Build history of the part. All positions in model axes, mm. A direction names the side the tool comes from. Give positions to 0.01 mm unless a question says otherwise; leave off trailing zeros. Loops run counter-clockwise (first coordinate to the right, second up) from the corner with the lowest first, then second, coordinate; pieces in that order, holes last. Notation, with made-up numbers: (-3.5, 39) - (28.5, 39) arc R31 ccw to (28.5, 66) - close; hole circle Ø8 at (22, 8.25). An arc over 180 degrees is marked (long way). Return JSON: item names as keys, results as strings. Group by question number.
1) Slice it at B-B (x = 40). List the corners of the cut face in (y, z).
2) Slice it at A-A (z = 1). Count the separate pieces of the cut face and the enclosed holes in it, and give its area (3 significant figures).
3) Drill centre lines: probe 1 along X at (y, z) = (-6.5, -0.5); probe 2 along Y at (x, z) = (36, 2.25); probe 3 along Y at (x, z) = (6.5, 1.75). Where is each one in solid material? Low to high. Write a range as from..to.
4) Drop flat-ended pins along their axis: pin 1 (4.5 mm diameter, centred on x = 20.5, y = 0.5, fed in from -Z); pin 2 (5.5 mm diameter, centred on x = 66.5, y = 7, fed in from +Z) (3 decimals); pin 3 (6 mm diameter, centred on x = 32, z = -4, fed in from +Y); pin 4 (3 mm diameter, centred on x = 39, y = -5, fed in from +Z). Give the stop position or say it passes through.
5) 3-axis set-ups, long thin cutter, end or side, ignore diameter. For faces 4 (the face through (24.504, -7, -1)), 5 (the face through (65, 6, -2.125)), 6 (the face through (65, 9.75, -3)), 7 (the face through (65, 2.16, -3)), 8 (the face through (0, 0, -7)): which of +Z, -Z, +X, -X, +Y, -Y reach the whole face in a straight line?
6) Slice it at D-D (z = -9.25). List the corners of the cut face in (x, y).
7) Mould opens along Y. For faces 1 (the face through (13.1, -17.5, 3)), 2 (the face through (38, -18.25, -2)), 3 (the face through (65, -3.3, -3)) say: released by +Y, released by -Y, zero draft, split by the parting line, or undercut.
```python
from build123d import *

# Parameters (mm, degrees)
SKETCH1_R               = 5.35
BOSS_EXTRUDE2_DEPTH     = 7
BOSS_EXTRUDE3_START     = 8
SKETCH3_R               = 5.35
BOSS_EXTRUDE3_DEPTH     = 8
BOSS_EXTRUDE4_DEPTH     = 3
CHAMFER1_SIZE           = 10
CHAMFER2_SIZE           = 5
CUT_EXTRUDE1_DEPTH      = 67.560662475
CUT_EXTRUDE1_DEPTH_BACK = 67.560662475
SKETCH5_W               = 31.474956737
SKETCH5_H               = 3.5
SKETCH5_H_2             = 8
CHAMFER3_SIZE           = 7
SKETCH6_W               = 2.75
SKETCH6_H               = 7.59
SKETCH6_H_2             = 11.2
BOSS_EXTRUDE5_DEPTH     = 5
SKETCH7_R               = 11
BOSS_EXTRUDE6_DEPTH     = 5
CUT_EXTRUDE2_REACH      = 87.717
SKETCH8_W               = 8
SKETCH8_H               = 4
SKETCH9_R               = 3.1
CUT_EXTRUDE3_DEPTH      = 4
CUT_EXTRUDE4_START      = -1
SKETCH10_R              = 3.1
CUT_EXTRUDE4_DEPTH      = 1
CHAMFER4_SIZE           = 1
FILLET3_R               = 0.5


# Some blends are built 0.0001 mm under size
with BuildPart() as part:
    # Sketch1 → Boss-Extrude2 (new body)
    with BuildSketch(Plane.XY):
        Polygon((-19.503784034, -20), (19.503784034, -20), (19.503784034, -18.25), (62.978740771, -18.25), (62.978740771, 13), (19.503784034, 13), (19.503784034, 20), (-19.503784034, 20), align=None)
        Circle(SKETCH1_R, mode=Mode.SUBTRACT)
    extrude(amount=-BOSS_EXTRUDE2_DEPTH)

    # Sketch3 → Boss-Extrude3 (add)
    with BuildSketch(Plane.XY.offset(BOSS_EXTRUDE3_START)):
        with BuildLine():
            Line((7.668115805, 5.35), (62.978740771, 5.35))
            Line((62.978740771, 5.35), (62.978740771, 9.35))
            Line((62.978740771, 9.35), (0, 9.35))
            ThreePointArc((0, 9.35), (-9.35, 0), (0, -9.35))
            Line((0, -9.35), (62.978740771, -9.35))
            Line((62.978740771, -9.35), (62.978740771, -5.35))
            Line((62.978740771, -5.35), (7.668115805, -5.35))
            ThreePointArc((7.668115805, -5.35), (9.35, 0), (7.668115805, 5.35))
        make_face()
        Circle(SKETCH3_R, mode=Mode.SUBTRACT)
    extrude(amount=-BOSS_EXTRUDE3_DEPTH)

    # Sketch4 → Boss-Extrude4 (add)
    with BuildSketch(Plane.XY):
        with BuildLine():
            Line((0, -18.25), (62.978740771, -18.25))
            Line((62.978740771, -18.25), (62.978740771, -17.25))
            Line((62.978740771, -17.25), (8.306623863, -17.25))
            Line((8.306623863, -17.25), (0, -17.25))
            ThreePointArc((0, -17.25), (-17.25, 0), (0, 17.25))
            Line((0, 17.25), (0, 18.25))
            ThreePointArc((0, 18.25), (-18.25, 0), (0, -18.25))
        make_face()
    extrude(amount=BOSS_EXTRUDE4_DEPTH)

    # Chamfer1
    # the kernel refuses this chamfer: 10 mm, written as the material it takes off along each edge
    with BuildSketch(Plane(origin=(19.503784034, -20, 25.71682988), x_dir=(-0.9996219169112968, -0.027495876610586317, 0), z_dir=(0, 0, -1))) as chamfer1_piece_1_section:
        Polygon((CHAMFER1_SIZE * 0.999621916911, CHAMFER1_SIZE * 0.0274958766106), (-CHAMFER1_SIZE * 0.0274958766106, CHAMFER1_SIZE * 0.999621916911), (0, 0), align=None)
    chamfer1_piece_1 = extrude(amount=58.433659759, mode=Mode.PRIVATE)
    chamfer1_piece_1 = split(chamfer1_piece_1, bisect_by=Plane(origin=(14.814200223, -18.25, -3.5), z_dir=(0, -1, 0)), keep=Keep.TOP, mode=Mode.PRIVATE)
    add(chamfer1_piece_1, mode=Mode.SUBTRACT)

    # Chamfer2
    chamfer2_edges = [part.edges().sort_by_distance(p)[0] for p in [
        (-19.503784034, -20, -3.5),
        (-19.503784034, 20, -3.5),
    ]]
    chamfer(chamfer2_edges, length=CHAMFER2_SIZE)

    # Sketch5 → Cut-Extrude1 (cut, two sides: drawn at the far end of the back side and taken through both)
    with BuildSketch(Plane.XY.offset(-CUT_EXTRUDE1_DEPTH_BACK)):
        with Locations((40.241262403, 3.6)):
            Rectangle(SKETCH5_W, SKETCH5_H)
        with Locations((40.241262403, -7.15)):
            Rectangle(SKETCH5_W, SKETCH5_H_2)
    extrude(amount=CUT_EXTRUDE1_DEPTH + CUT_EXTRUDE1_DEPTH_BACK, mode=Mode.SUBTRACT)

    # Chamfer3
    chamfer3_edges = [part.edges().sort_by_distance(p)[0] for p in [
        (19.503784034, 20, -3.5),
    ]]
    chamfer(chamfer3_edges, length=CHAMFER3_SIZE - 0.0001)  # a hair under: the kernel refuses the full size

    # Sketch6 → Boss-Extrude5 (add)
    with BuildSketch(Plane(origin=(62.978740771, 0, 0), x_dir=(0, 0, -1), z_dir=(1, 0, 0))):
        with Locations((3.5, 5.955)):
            Rectangle(SKETCH6_W, SKETCH6_H)
        with Locations((3.5, -8.9)):
            Rectangle(SKETCH6_W, SKETCH6_H_2)
    extrude(amount=BOSS_EXTRUDE5_DEPTH)

    # Sketch7 → Boss-Extrude6 (add)
    with BuildSketch(Plane(origin=(0, 0, -7), x_dir=(-1, 0, 0), z_dir=(0, 0, -1))):
        Circle(SKETCH7_R)
    extrude(amount=BOSS_EXTRUDE6_DEPTH)

    # Sketch8 → Cut-Extrude2 (cut, up to next)
    with BuildSketch(Plane(origin=(62.978740771, 0, 0), x_dir=(0, 0, -1), z_dir=(1, 0, 0)), mode=Mode.PRIVATE) as cut_extrude2_sk1:
        with Locations((-4, -7.35)):
            Rectangle(SKETCH8_W, SKETCH8_H)
    cut_extrude2_tool1 = extrude(cut_extrude2_sk1.sketch, amount=-CUT_EXTRUDE2_REACH, mode=Mode.PRIVATE) & part.part
    add(cut_extrude2_tool1.solids().sort_by_distance((62.978741, -7.35, 4))[0], mode=Mode.SUBTRACT)

    # Sketch9 → Cut-Extrude3 (cut)
    with BuildSketch(Plane.XY):
        with Locations((20.003784034, 0)):
            Circle(SKETCH9_R)
    extrude(amount=-CUT_EXTRUDE3_DEPTH, mode=Mode.SUBTRACT)

    # Sketch10 → Cut-Extrude4 (cut)
    with BuildSketch(Plane(origin=(0, 0, -7), x_dir=(-1, 0, 0), z_dir=(0, 0, -1)).offset(CUT_EXTRUDE4_START)):
        with Locations(Location((-20.003784034, 0, 0), (0, 0, 180))):
            Circle(SKETCH10_R)
    extrude(amount=CUT_EXTRUDE4_DEPTH, mode=Mode.SUBTRACT)

    # Chamfer4
    chamfer4_edges = [part.edges().sort_by_distance(p)[0] for p in [
        (16.903784034, 0, -6),
    ]]
    chamfer(chamfer4_edges, length=CHAMFER4_SIZE - 0.0001)  # a hair under: the kernel refuses the full size

    # Fillet3
    fillet3_edges = [part.edges().sort_by_distance(p)[0] for p in [
        (0, 18.25, 1.5),
        (0, 17.25, 1.5),
    ]]
    fillet(fillet3_edges, radius=FILLET3_R - 0.0001)  # a hair under: the kernel refuses the full size


solid = part.part
```
Results:
{
 "1": {"outline": "(-18.25, -7) - (-11.15, -7) - (-11.15, 0) - (-17.25, 0) - (-17.25, 3) - (-18.25, 3) - close; (-3.15, -7) - (1.85, -7) - (1.85, 0) - (-3.15, 0) - close; (5.35, -7) - (13, -7) - (13, 0) - (9.35, 0) - (9.35, 8) - (5.35, 8) - close"},
 "2": {"separate pieces": "2", "enclosed holes": "1", "area": "610 mm2"},
 "3": {"probe 1": "-19.5..24.5, 55.98..62.98", "probe 2": "-18.25..-17.25, 5.35..9.35", "probe 3": "-18.25..-17.25, -9.35..9.35"},
 "4": {"pin 1": "z = -6.85", "pin 2": "z = -2.125", "pin 3": "y = 13", "pin 4": "through"},
 "5": {"face 4": "+Z, -Z", "face 5": "+Z, +X, +Y, -Y", "face 6": "+Z, -Z, +X, +Y", "face 7": "+Z, -Z, +X", "face 8": "+Z"},
 "6": {"outline": "circle Ø22 at (0, 0)"},
 "7": {"face 1": "zero draft", "face 2": "released by -Y", "face 3": "undercut"}
}
